For this review, use the dimensioned drawing (mm, ordinates from the lowest corner) and the shaded views. A direction names the side the tool comes from. Give positions to 0.01 mm unless a question says otherwise; leave off trailing zeros. Order: outer loops, then holes, each group sorted by start corner. A loop starts at its lowest first (then second) coordinate and runs counter-clockwise, first axis right, second up.
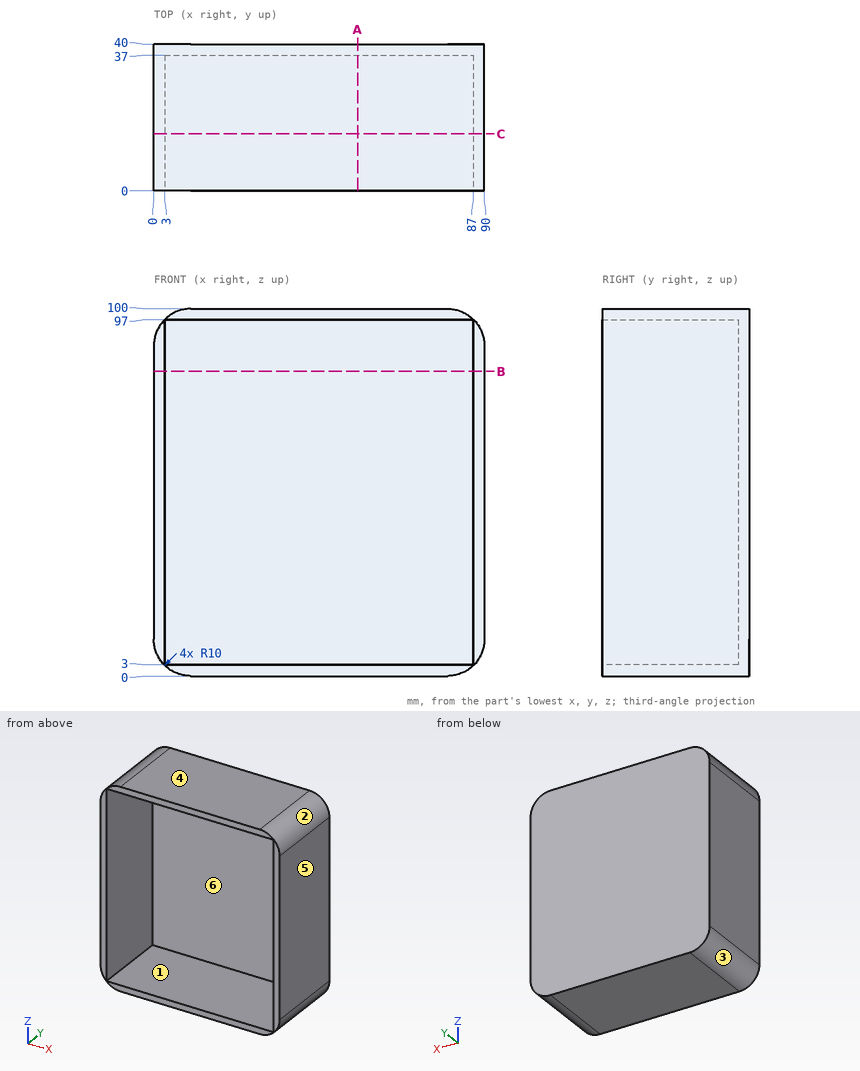
1. Take a section at C-C (y = 15.5). State the section outline as (x, z) points, then the cut area to 3 significant figures.
Recorded:
outline: (0, 10) arc R10 ccw to (10, 0) - (80, 0) arc R10 ccw to (90, 10) - (90, 90) arc R10 ccw to (80, 100) - (10, 100) arc R10 ccw to (0, 90) - close; hole (3, 3) - (87, 3) - (87, 97) - (3, 97) - close
area: 1,020 mm2
2. Machinability: for the marked faces 1 and 2, which of the approach directions +Z, -Z, +X, -X, +Y, -Y give a long, thin tool a straight path to every point of the face, cutting with its end or side? Answer none if there is none.
Recorded:
face 1: -Y
face 2: +Z, +X, +Y, -Y
3. For pin 1 (8 mm diameter, centred on x = 42.5, z = 49, fed in from -Y), flat-tipped, find the tip position at first contact; note if it passes through.
Recorded:
pin 1: stops at y = 37
4. Draft analysis for pull direction X (two halves, no side actions). For the marked faces 3, 4, 5 and 6, state which applies: pulls with the +X half, pulls with the -X half, needs draft (parallel to the pull), parting line crosses it, or undercut.
Recorded:
face 3: pulls with the -X half
face 4: needs draft
face 5: pulls with the +X half
face 6: undercut
5. For line 1 along Z through (x, y) = (34, 3); line 2 along X through (y, z) = (2.5, 55); line 3 along Y through (x, z) = (48.5, 66), list the stretches that pass through material, from the lowest coordinate up.
Recorded:
line 1: z = 0 to 3, 97 to 100
line 2: x = 0 to 3, 87 to 90
line 3: y = 37 to 40
6. Take a section at B-B (z = 83). State the section outline as (x, y) points.
Recorded:
outline: (0, 0) - (3, 0) - (3, 37) - (87, 37) - (87, 0) - (90, 0) - (90, 40) - (0, 40) - close
7. Take a section at A-A (x = 55.5). State the section outline as (y, z) points.
Recorded:
outline: (0, 0) - (40, 0) - (40, 100) - (0, 100) - (0, 97) - (37, 97) - (37, 3) - (0, 3) - close
